Model file for the job. Use its own axes, mm. A direction names the side the tool comes from. Coordinates: 2 decimals unless noted, no trailing zeros. Order: outer loops, then holes, each group sorted by start corner. A loop starts at its lowest first (then second) coordinate and runs counter-clockwise, first axis right, second up.
from build123d import *

# Parameters (mm, degrees)
SKETCH1_R           = 1.8
SKETCH1_W           = 5
SKETCH1_H           = 20
BOSS_EXTRUDE1_DEPTH = 5.08


with BuildPart() as part:
    # Sketch1 → Boss-Extrude1 (new body)
    with BuildSketch(Plane(origin=(0, 0, 0), x_dir=(0, 1, 0), z_dir=(0, 0, 1))):
        Polygon((-41.181536726, 53.881536726), (-19.05, 53.881536726), (-12.7, 60.231536726), (12.7, 60.231536726), (19.05, 53.881536726), (41.181536726, 53.881536726), (53.881536726, 41.181536726), (53.881536726, 19.05), (60.231536726, 12.7), (60.231536726, -12.7), (53.881536726, -19.05), (53.881536726, -41.181536726), (41.181536726, -53.881536726), (19.05, -53.881536726), (12.7, -60.231536726), (-12.7, -60.231536726), (-19.05, -53.881536726), (-41.181536726, -53.881536726), (-53.881536726, -41.181536726), (-53.881536726, -19.05), (-60.231536726, -12.7), (-60.231536726, 12.7), (-53.881536726, 19.05), (-53.881536726, 41.181536726), align=None)
        with Locations((-46.633511114, -37.653254993)):
            Circle(SKETCH1_R, mode=Mode.SUBTRACT)
        with Locations((-37.653254993, -46.633511114)):
            Circle(SKETCH1_R, mode=Mode.SUBTRACT)
        with Locations((46.633511114, -37.653254993)):
            Circle(SKETCH1_R, mode=Mode.SUBTRACT)
        with Locations((37.653254993, -46.633511114)):
            Circle(SKETCH1_R, mode=Mode.SUBTRACT)
        with Locations((-46.633511114, 37.653254993)):
            Circle(SKETCH1_R, mode=Mode.SUBTRACT)
        with Locations((-37.653254993, 46.633511114)):
            Circle(SKETCH1_R, mode=Mode.SUBTRACT)
        with Locations((37.653254993, 46.633511114)):
            Circle(SKETCH1_R, mode=Mode.SUBTRACT)
        with Locations((46.633511114, 37.653254993)):
            Circle(SKETCH1_R, mode=Mode.SUBTRACT)
        with Locations((-22.86, -16.51)):
            Circle(SKETCH1_R, mode=Mode.SUBTRACT)
        with Locations((22.86, -16.51)):
            Circle(SKETCH1_R, mode=Mode.SUBTRACT)
        with Locations((22.86, 29.21)):
            Circle(SKETCH1_R, mode=Mode.SUBTRACT)
        with Locations((-22.86, 29.21)):
            Circle(SKETCH1_R, mode=Mode.SUBTRACT)
        with Locations((9.525, -56.421536726)):
            Circle(SKETCH1_R, mode=Mode.SUBTRACT)
        with Locations((-9.525, -56.421536726)):
            Circle(SKETCH1_R, mode=Mode.SUBTRACT)
        with Locations((-56.421536726, -9.525)):
            Circle(SKETCH1_R, mode=Mode.SUBTRACT)
        with Locations((-56.421536726, 9.525)):
            Circle(SKETCH1_R, mode=Mode.SUBTRACT)
        with Locations((-9.525, 56.421536726)):
            Circle(SKETCH1_R, mode=Mode.SUBTRACT)
        with Locations((9.525, 56.421536726)):
            Circle(SKETCH1_R, mode=Mode.SUBTRACT)
        with Locations((56.421536726, 9.525)):
            Circle(SKETCH1_R, mode=Mode.SUBTRACT)
        with Locations((56.421536726, -9.525)):
            Circle(SKETCH1_R, mode=Mode.SUBTRACT)
        with Locations((-30, 0)):
            Rectangle(SKETCH1_W, SKETCH1_H, mode=Mode.SUBTRACT)
        with Locations((30, 0)):
            Rectangle(SKETCH1_W, SKETCH1_H, mode=Mode.SUBTRACT)
    extrude(amount=BOSS_EXTRUDE1_DEPTH)


solid = part.part
Q1. Probe line 1 (X direction, y = 23, z = 3.65); line 2 (X direction, y = 38, z = 4.2); line 3 (Y direction, x = 6, z = 0.3). List the from-to ranges inside material, lowest first.
Established:
line 1: x = -53.88 to -31, -27.42 to 14.72, 18.3 to 53.88
line 2: x = -53.88 to -48.4, -44.87 to 44.87, 48.4 to 53.88
line 3: y = -60.23 to -32.5, -27.5 to 27.5, 32.5 to 60.23
Q2. Cut at D-D, the plane z = 2.45. Count the separate pieces of the cut face and the enclosed holes in it, plus the area to 3 significant figures.
Established:
separate pieces: 1
enclosed holes: 22
area: 11,700 mm2
Q3. Mould opens along X. For faces 6 (the face through (-57.01, -15.92, 2.5)), 7 (the face through (10, -30, 3)), 8 (the face through (53.882, 30, 3)) say: pulls with the +X half, pulls with the -X half, needs draft (parallel to the pull), parting line crosses it, or undercut.
Established:
face 6: pulls with the -X half
face 7: undercut
face 8: pulls with the +X half
Q4. Cut at B-B, the plane y = -22.86. List the corners of the cut face in (x, z), plus the area to 3 significant figures.
Established:
outline: (-53.88, 0) - (-31.01, 0) - (-31.01, 5.08) - (-53.88, 5.08) - close; (-27.41, 0) - (14.71, 0) - (14.71, 5.08) - (-27.41, 5.08) - close; (18.31, 0) - (53.88, 0) - (53.88, 5.08) - (18.31, 5.08) - close
area: 511 mm2
Q5. Cut at A-A, the plane x = -29.21. List the corners of the cut face in (y, z).
Established:
outline: (-53.88, 0) - (-24.66, 0) - (-24.66, 5.08) - (-53.88, 5.08) - close; (-21.06, 0) - (21.06, 0) - (21.06, 5.08) - (-21.06, 5.08) - close; (24.66, 0) - (53.88, 0) - (53.88, 5.08) - (24.66, 5.08) - close
Q6. Drop flat-ended pins along their axis: P1, Ø2, axis at x = 37.65, y = 46.63, coming from the -Z side; P2, Ø1.5, axis at y = -29, z = 3, coming from the -X side; P3, Ø2, axis at x = -15.5, z = 1, coming from the -Y side; P4, Ø1.5, axis at x = -27, z = 3.5, coming from the +Y side. Give the stop position or say it passes through.
Established:
P1: passes through
P2: stops at x = -53.88
P3: stops at y = -58.43
P4: stops at y = 53.88
Q7. Which spindle directions (+Z, -Z, +X, -X, +Y, -Y) get a long thin tool onto all of the face, cutting with end or side? Do faces 1 (the face through (-30, -53.882, 3)), 2 (the face through (-53.882, 30, 3)), 3 (the face through (30, 53.882, 3)), 4 (the face through (0, -32.5, 3)), 5 (the face through (0, 60.232, 3)). Say none if no direction does.
Established:
face 1: +Z, -Z, -X, -Y
face 2: +Z, -Z, -X, +Y
face 3: +Z, -Z, +X, +Y
face 4: +Z, -Z
face 5: +Z, -Z, +X, -X, +Y
Q8. Cut at C-C, the plane x = 28.5. List the corners of the cut face in (y, z).
Established:
outline: (-53.88, 0) - (53.88, 0) - (53.88, 5.08) - (-53.88, 5.08) - close
